Work out the finished part from the listing and answer in its coordinate system (mm). A direction names the side the tool comes from. Give positions to 0.01 mm unless a question says otherwise; leave off trailing zeros. Write each loop counter-clockwise with the first axis right and the second up, starting at its lowest first coordinate (ties: lowest second). Pieces come first, ordered by that corner, then holes.
1) Given pin 1 Ø1.2 at (x, y) = (-0.5, 17) entering from +Z; pin 2 Ø5 at (x, z) = (0, -38) entering from +Y; pin 3 Ø6 at (x, z) = (-1, -74.5) entering from -Y, each flat-ended and moving along its own axis, determine where each tip first touches the part or whether it passes through.
2) Straight lines are drawn through the part: probe 1 along Z at (x, y) = (20.5, 4); probe 2 along Z at (x, y) = (-10.5, -4.5); probe 3 along Y at (x, z) = (0, -25.5). For each, find the intervals that lie inside material, in ascending order.
3) Find section B-B (z = -120). Determine the outline of the cut face in (x, y), plus the area to 3 significant figures.
4) Find section C-C (z = -70.5). Determine the outline of the cut face in (x, y).
5) Find section D-D (z = -47). Determine the outline of the cut face in (x, y).
6) Determine the mould class of faces 1 (the face through (-10, 14, -88)), 2 (the face through (15.9, -1.2, -3)), 3 (the face through (-18, 0, -6)) for opening direction Z: pulls with the +Z half, pulls with the -Z half, needs draft (parallel to the pull), parting line crosses it, or undercut.
7) Find section A-A (y = 29.5). Determine the outline of the cut face in (x, z), plus the area to 3 significant figures.
8) A tool of negligible diameter and unlimited length cuts with its end or side. For faces 4 (the face through (2, 22, -116)), 5 (the face through (-14, 10, -88)), 6 (the face through (-0.812, -23.236, -130.05)), 7 (the face through (10, 14, -88)), 8 (the face through (-0.867, -3.905, -20.678)), from which of +Z, -Z, +X, -X, +Y, -Y can it reach the whole face along a straight path? Write none if from no direction.
Autodesk Inventor part; units mm, degrees
ref_plane "YZ Plane" through (0, 0, 0) normal (1, 0, 0) x (0, 1, 0)
ref_plane "XY Plane" through (0, 0, 0) normal (0, 0, 1) x (1, 0, 0)
sketch "Sketch1" plane through (0, 0, 0) normal (0, 0, 1) x (1, 0, 0)
  circle A0 centre (0, 0) radius 20.85
  dimension "d0" = 41.7
extrude "Extrusion1" add sketch "Sketch1" against normal blind 116
ref_plane "Work Plane3" through (0, 0, -44) normal (0, 0, -1) x (-1, 0, 0)
ref_plane "Work Plane2" through (0, 0, -52) normal (0, 0, -1) x (-1, 0, 0)
sketch "Sketch2" plane through (0, 0, -84) normal (0, 0, -1) x (-1, 0, 0)
  circle A0 centre (0, 0) radius 20.85
  circle A1 centre (0, 0) radius 21
  dimension "d6" = 42
extrude "Extrusion2" add sketch "Sketch2" along normal up to surface (32 mm away)
sketch "Sketch3" plane through (0, 0, -84) normal (0, 0, -1) x (-1, 0, 0)
  circle A0 centre (0, 0) radius 22
  circle A1 centre (0, 0) radius 20.85
  dimension "d9" = 44
extrude "Extrusion3" add sketch "Sketch3" against normal up to surface (32 mm away)
sketch "Sketch4" plane through (0, 0, 0) normal (0, 0, 1) x (1, 0, 0)
  circle A0 centre (0, 0) radius 17.5
  circle A1 centre (0, 17.5) radius 2
  circle A2 centre (-17.5, 0) radius 2
  circle A3 centre (0, -17.5) radius 2
  circle A4 centre (17.5, 0) radius 2
  dimension "d12" = 35
  dimension "d13" = 4
  dimension "d16" = 360
extrude "Extrusion4" cut sketch "Sketch4" against normal blind 6 contours A0 A4 | A0 A4 | A1 A0 | A0 A1 | A3 A0 | A0 A3 | A2 A0 | A0 A2
sketch "Sketch5" plane through (0, 0, 0) normal (0, 0, 1) x (1, 0, 0)
  circle A0 centre (0, 0) radius 12.5
  dimension "d20" = 25
extrude "Extrusion5" add sketch "Sketch5" along normal blind 2
sketch "Sketch6" plane through (0, 0, 2) normal (0, 0, 1) x (1, 0, 0)
  circle A0 centre (0, 0) radius 4
  dimension "d23" = 8
extrude "Extrusion6" cut sketch "Sketch6" against normal up to surface (46 mm away)
sketch "Sketch7" plane through (0, 0, -116) normal (0, 0, -1) x (-1, 0, 0)
  circle A0 centre (0, 0) radius 23.25
  circle A1 centre (0, 0) radius 21
  dimension "d26" = 46.5
  dimension "d27" = 42
extrude "Extrusion7" add sketch "Sketch7" along normal blind 28.5 contours A0 | A1
ref_plane "Work Plane4" through (0, 17.5, 0) normal (0, 1, 0) x (-1, 0, 0)
sketch "Sketch8" plane through (0, 17.5, 0) normal (0, 1, 0) x (-1, 0, 0)
  line L0 (-23.25, -144.5) -> (23.25, -144.5)
  line L1 (-23.25, -116) -> (23.25, -116)
  line L2 (-23.25, -116) -> (23.25, -116)
  line L3 (-23.25, -144.5) -> (23.25, -144.5)
  line L4 (23.25, -116) -> (-23.25, -144.5)
  line L5 (-14, -116) -> (14, -116)
  line L6 (14, -116) -> (14, -144.5)
  line L7 (14, -144.5) -> (-14, -144.5)
  line L8 (-14, -144.5) -> (-14, -116)
  line L9 (-14, -116) -> (14, -144.5) construction
  line L10 (14, -116) -> (-14, -144.5) construction
  point P0 (0, 0)
  point P1 (0, -130.25)
  dimension "d31" = 28
extrude "Extrusion8" add sketch "Sketch8" along normal blind 21.5 contours L8 L4 L6 L0 | L8 L1 L6 L4
ref_plane "Work Plane5" through (0, 0, -42) normal (0, 0, 1) x (1, 0, 0)
ref_plane "Work Plane6" through (0, 0, -10) normal (0, 0, 1) x (1, 0, 0)
sketch "Sketch9" plane through (0, 0, -10) normal (0, 0, 1) x (1, 0, 0)
  circle A0 centre (0, 0) radius 12.5
  circle A1 centre (-17.5, 0) radius 2
  circle A2 centre (0, 17.5) radius 2
  circle A3 centre (0, -17.5) radius 2
  circle A4 centre (17.5, 0) radius 2
  circle A5 centre (0, 0) radius 20.85
  circle A6 centre (0, 0) radius 4
  circle A7 centre (0, 0) radius 21.35
  dimension "d36" = 42.7
extrude "Extrusion9" add sketch "Sketch9" against normal up to surface (32 mm away) contours A7
ref_plane "Work Plane7" through (0, 21, 0) normal (0, 1, 0) x (-1, 0, 0)
sketch "Sketch10" plane through (0, 21, 0) normal (0, 1, 0) x (-1, 0, 0)
  line L0 (-21, -84) -> (21, -84)
  line L1 (-21, -116) -> (21, -116)
  line L2 (-21, -84) -> (21, -84)
  line L3 (0, -84) -> (0, -88)
  line L4 (-10, -90) -> (10, -90)
  line L5 (10, -90) -> (10, -86)
  line L6 (10, -86) -> (-10, -86)
  line L7 (-10, -86) -> (-10, -90)
  line L8 (-10, -90) -> (10, -86) construction
  line L9 (10, -90) -> (-10, -86) construction
  point P0 (0, 0)
  dimension "d40" = 4
  dimension "d41" = 20
  dimension "d42" = 4
extrude "Extrusion10" cut sketch "Sketch10" against normal through all
pattern_circular "Circular Pattern1" count 2 over 90 about axis through (0, 0, -84) along (0, 0, -1) of "Extrusion10"
thread "Thread1"
thread "Thread2"
thread "Thread3"
thread "Thread4"
ref_plane "Work Plane1" through (0, 0, -84) normal (0, 0, -1) x (-1, 0, 0)
properties part number "motorbody"
Results:
1. pin 1: stops at z = -6
1. pin 2: stops at y = 21.35
1. pin 3: stops at y = -22
2. probe 1: z = -144.5 to -90, -86 to -52, -42 to -10
2. probe 2: z = -144.5 to -90, -86 to 2
2. probe 3: y = -21.35 to -4, 4 to 21.35
3. outline: (-14, 18.56) arc R23.25 ccw (long way) to (14, 18.56) - (14, 39) - (-14, 39) - close
3. area: 2,180 mm2
4. outline: circle Ø44 at (0, 0)
5. outline: circle Ø41.7 at (0, 0)
6. face 1: undercut
6. face 2: needs draft
6. face 3: pulls with the +Z half
7. outline: (-14, -144.5) - (14, -144.5) - (14, -116) - (-14, -116) - close
7. area: 798 mm2
8. face 4: none
8. face 5: +X, -X
8. face 6: +Z, -Z
8. face 7: +Y, -Y
8. face 8: +Z
